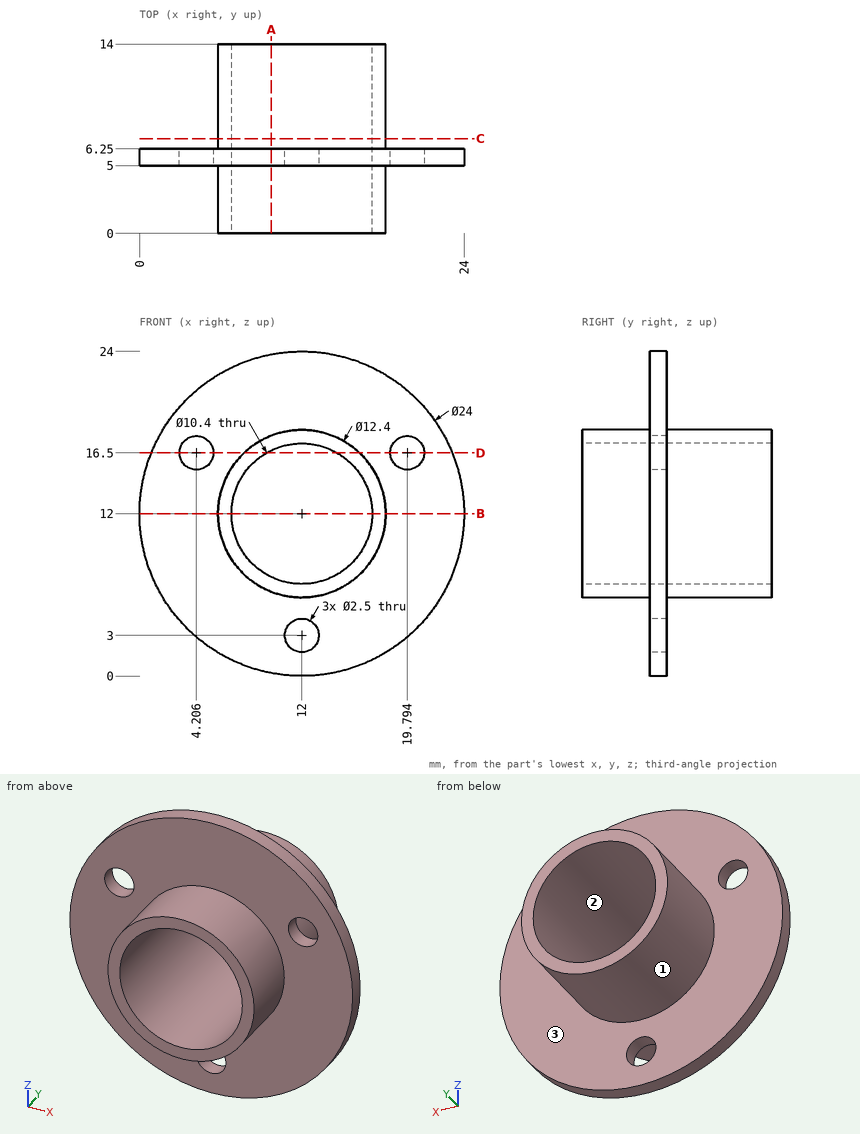
Check sheet for the drawn part. Datum: minimum x, y, z corner. Units: mm. Coordinates: 2 decimals unless noted, no trailing zeros. Loops run counter-clockwise (first coordinate to the right, second up) from the corner with the lowest first, then second, coordinate; pieces in that order, holes last. Notation, with made-up numbers: (36.25, 29.5) -> (77.25, 29.5) arc R5 ccw to (77.25, 33.5) -> close; hole circle Ø3 at (18.5, -3.5). An arc over 180 degrees is marked (long way). Answer in a Markdown table with one row per item.
1) Scan lines: line 1 along X through (y, z) = (4.75, 12); line 2 along Y through (x, z) = (14.25, 22.25); line 3 along X through (y, z) = (3, 15) (1 decimal). Record each from-to range of solid material in increasing order. Write a range as from..to.
The answers:
| item | result |
|---|---|
| line 1 | x = 5.8..6.8, 17.2..18.2 |
| line 2 | y = 5..6.25 |
| line 3 | x = 6.6..7.8, 16.2..17.4 |
2) Section check C-C (y = 7). Record the cut outline in (x, z).
The answers:
| item | result |
|---|---|
| outline | circle Ø12.4 at (12, 12); hole circle Ø10.4 at (12, 12) |
3) Depth check by flat-ended pin: P1, Ø4, axis at x = 12, z = 3, coming from the +Y side; P2, Ø5, axis at y = 10.5, z = 16.5, coming from the +X side; P3, Ø4, axis at x = 6.5, y = 6.5, coming from the -Z side. Enter the tip coordinate at first touch or a pass-through.
The answers:
| item | result |
|---|---|
| P1 | stops at y = 6.25 |
| P2 | stops at x = 17.87 |
| P3 | stops at z = 0.53 |
4) Draft check along Z on the marked faces 1, 2 and 3. Enter one of: released by +Z, released by -Z, zero draft, split by the parting line, or undercut.
The answers:
| item | result |
|---|---|
| face 1 | split by the parting line |
| face 2 | undercut |
| face 3 | zero draft |
5) Section check A-A (x = 9.75). Record the cut outline in (y, z).
The answers:
| item | result |
|---|---|
| outline | (0, 6.22) -> (5, 6.22) -> (5, 0.21) -> (6.25, 0.21) -> (6.25, 6.22) -> (14, 6.22) -> (14, 7.31) -> (0, 7.31) -> close; (0, 16.69) -> (14, 16.69) -> (14, 17.78) -> (6.25, 17.78) -> (6.25, 23.79) -> (5, 23.79) -> (5, 17.78) -> (0, 17.78) -> close |
6) Section check D-D (z = 16.5). Give the number of separate pieces and of enclosed holes in the cut face.
The answers:
| item | result |
|---|---|
| separate pieces | 4 |
| enclosed holes | 0 |
7) Section check B-B (z = 12). Record the cut outline in (x, y).
The answers:
| item | result |
|---|---|
| outline | (0, 5) -> (5.8, 5) -> (5.8, 0) -> (6.8, 0) -> (6.8, 14) -> (5.8, 14) -> (5.8, 6.25) -> (0, 6.25) -> close; (17.2, 0) -> (18.2, 0) -> (18.2, 5) -> (24, 5) -> (24, 6.25) -> (18.2, 6.25) -> (18.2, 14) -> (17.2, 14) -> close |
